For this review, take the finished solid that the model builds, in its own axes (mm). Face numbers are marked on the shaded views. A direction names the side the tool comes from. Give positions to 0.01 mm unless a question says otherwise; leave off trailing zeros. Loops run counter-clockwise (first coordinate to the right, second up) from the corner with the lowest first, then second, coordinate; pieces in that order, holes last. Notation, with made-up numbers: (41.25, 3.5) - (62.25, 3.5) arc R20 cw to (62.25, 10.5) - close; hole circle Ø7 at (39, 1.25). An arc over 180 degrees is marked (long way). Answer as CSV lines item,"result".
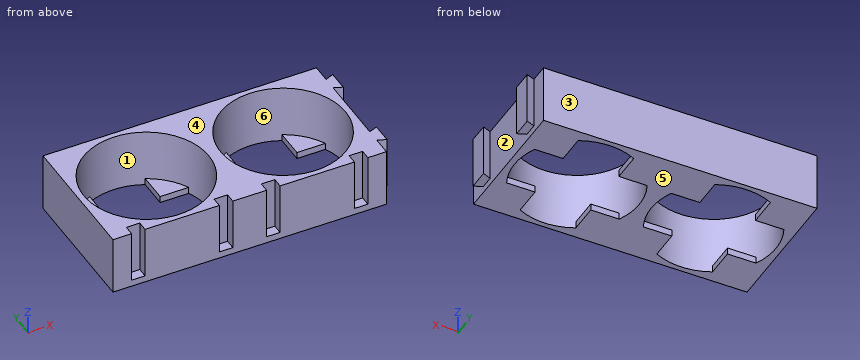
from build123d import *

# Parameters (mm, degrees)
SKETCH1_W           = 40.5
SKETCH1_H           = 20
SKETCH1_R           = 9.25
BOSS_EXTRUDE1_DEPTH = 8.8
SKETCH2_W           = 2
SKETCH2_H           = 7.8
CUT_EXTRUDE1_DEPTH  = 1.5
BOSS_EXTRUDE2_DEPTH = 1


with BuildPart() as part:
    # Sketch1 → Boss-Extrude1 (new body)
    with BuildSketch(Plane.XY):
        Rectangle(SKETCH1_W, SKETCH1_H)
        with Locations((-10.125, 0)):
            Circle(SKETCH1_R, mode=Mode.SUBTRACT)
        with Locations((10.125, 0)):
            Circle(SKETCH1_R, mode=Mode.SUBTRACT)
    extrude(amount=BOSS_EXTRUDE1_DEPTH)

    # Sketch2 → Cut-Extrude1 (cut)
    with BuildSketch(Plane.XZ.offset(10)):
        with Locations((-16.5, 4.9)):
            Rectangle(SKETCH2_W, SKETCH2_H)
        with Locations((-3.5, 4.9)):
            Rectangle(SKETCH2_W, SKETCH2_H)
        with Locations((3.5, 4.9)):
            Rectangle(SKETCH2_W, SKETCH2_H)
        with Locations((16.5, 4.9)):
            Rectangle(SKETCH2_W, SKETCH2_H)
    extrude(amount=-CUT_EXTRUDE1_DEPTH, mode=Mode.SUBTRACT)

    # Sketch3 → Boss-Extrude2 (add)
    with BuildSketch(Plane(origin=(0, 0, 0), x_dir=(-1, 0, 0), z_dir=(0, 0, -1))):
        with BuildLine():
            Line((-14.25, 4), (-14.25, 8.279304017))
            ThreePointArc((-14.25, 8.279304017), (-16.714745453, 6.491360016), (-18.465413659, 4))
            Line((-18.465413659, 4), (-14.25, 4))
        make_face()
        with BuildLine():
            Line((-6, 4), (-1.784586341, 4))
            ThreePointArc((-1.784586341, 4), (-3.535254547, 6.491360016), (-6, 8.279304017))
            Line((-6, 8.279304017), (-6, 4))
        make_face()
        with BuildLine():
            ThreePointArc((-6, -8.279304017), (-3.535254547, -6.491360016), (-1.784586341, -4))
            Line((-1.784586341, -4), (-6, -4))
            Line((-6, -4), (-6, -8.279304017))
        make_face()
        with BuildLine():
            Line((-14.25, -4), (-18.465413659, -4))
            ThreePointArc((-18.465413659, -4), (-16.714745453, -6.491360016), (-14.25, -8.279304017))
            Line((-14.25, -8.279304017), (-14.25, -4))
        make_face()
        with BuildLine():
            Line((1.784586341, 4), (6, 4))
            Line((6, 4), (6, 8.279304017))
            ThreePointArc((6, 8.279304017), (3.535254547, 6.491360016), (1.784586341, 4))
        make_face()
        with BuildLine():
            ThreePointArc((18.465413659, 4), (16.714745453, 6.491360016), (14.25, 8.279304017))
            Line((14.25, 8.279304017), (14.25, 4))
            Line((14.25, 4), (18.465413659, 4))
        make_face()
        with BuildLine():
            Line((14.25, -4), (14.25, -8.279304017))
            ThreePointArc((14.25, -8.279304017), (16.714745453, -6.491360016), (18.465413659, -4))
            Line((18.465413659, -4), (14.25, -4))
        make_face()
        with BuildLine():
            Line((6, -4), (1.784586341, -4))
            ThreePointArc((1.784586341, -4), (3.535254547, -6.491360016), (6, -8.279304017))
            Line((6, -8.279304017), (6, -4))
        make_face()
    extrude(amount=-BOSS_EXTRUDE2_DEPTH)

    # Sketch4 → Loft1 section 0
    with BuildSketch(Plane(origin=(20.25, 0, 0), x_dir=(0, 0, -1), z_dir=(1, 0, 0))):
        with BuildLine():
            Line((-8.8, 7.25), (-1, 7.25))
            Line((-1, 7.25), (-1, 5.25))
            Line((-1, 5.25), (-8.8, 5.25))
            Line((-8.8, 5.25), (-8.8, 7.25))
        make_face()
    # Sketch5 → Loft1 section 1
    with BuildSketch(Plane(origin=(21.5, 0, 0), x_dir=(0, 0, -1), z_dir=(1, 0, 0))):
        with BuildLine():
            Line((-8.8, 7.75), (-1, 7.75))
            Line((-1, 7.75), (-1, 4.75))
            Line((-1, 4.75), (-8.8, 4.75))
            Line((-8.8, 4.75), (-8.8, 7.75))
        make_face()
    loft()

    # Sketch4<3> → Loft2 section 0
    with BuildSketch(Plane(origin=(20.25, 0, 0), x_dir=(0, 0, -1), z_dir=(1, 0, 0))):
        with BuildLine():
            Line((-8.8, -5.25), (-1, -5.25))
            Line((-1, -5.25), (-1, -7.25))
            Line((-1, -7.25), (-8.8, -7.25))
            Line((-8.8, -7.25), (-8.8, -5.25))
        make_face()
    # Sketch5<3> → Loft2 section 1
    with BuildSketch(Plane(origin=(21.5, 0, 0), x_dir=(0, 0, -1), z_dir=(1, 0, 0))):
        with BuildLine():
            Line((-8.8, -4.75), (-1, -4.75))
            Line((-1, -4.75), (-1, -7.75))
            Line((-1, -7.75), (-8.8, -7.75))
            Line((-8.8, -7.75), (-8.8, -4.75))
        make_face()
    loft()


solid = part.part
1) Machinability: for the marked faces 5 and 6, which of the approach directions +Z, -Z, +X, -X, +Y, -Y give a long, thin tool a straight path to every point of the face, cutting with its end or side? Answer none if there is none.
From the geometry:
face 5,"-Z, +X, -X, +Y, -Y"
face 6,"+Z"
2) Wall thickness on line 1 (X direction, y = 0, z = 4) (3 decimals); line 2 (Y direction, x = -17.5, z = 0.75); line 3 (Y direction, x = 10, z = 4.5): over which ranges is each line inside the solid? List them lowest first. Write a range as from..to.
From the geometry:
line 1,"x = -20.25..-19.375, -0.875..0.875, 19.375..20.25"
line 2,"y = -10..-4, 4..10"
line 3,"y = -10..-9.25, 9.25..10"
3) Consider section B-B on z = 5. Count the separate pieces of the cut face and the enclosed holes in it, and give its area (3 significant figures).
From the geometry:
separate pieces,"1"
enclosed holes,"2"
area,"267 mm^2"
4) Consider section D-D on x = 7. Write out the cut boundary in (y, z), and give its area (3 significant figures).
From the geometry:
outline,"(-10, 0) - (-8.71, 0) - (-8.71, 8.8) - (-10, 8.8) - close; (8.71, 0) - (10, 0) - (10, 8.8) - (8.71, 8.8) - close"
area,"22.8 mm^2"
5) Consider section C-C on x = 11.5. Write out the cut boundary in (y, z).
From the geometry:
outline,"(-10, 0) - (-9.15, 0) - (-9.15, 8.8) - (-10, 8.8) - close; (9.15, 0) - (10, 0) - (10, 8.8) - (9.15, 8.8) - close"
6) Consider section A-A on y = 0. Write out the cut boundary in (x, z) (3 decimals).
From the geometry:
outline,"(-20.25, 0) - (-19.375, 0) - (-19.375, 8.8) - (-20.25, 8.8) - close; (-0.875, 0) - (0.875, 0) - (0.875, 8.8) - (-0.875, 8.8) - close; (19.375, 0) - (20.25, 0) - (20.25, 8.8) - (19.375, 8.8) - close"
7) Insertion check: P1, Ø1.2, axis at y = -9, z = 5, coming from the +X side. The pin has a flat end and moves straight along its axis. Give the tip position at first contact, or say it passes through.
From the geometry:
P1,"stops at x = 20.25"
8) Draft analysis for pull direction Y (two halves, no side actions). For the marked faces 1, 2, 3 and 4, state which applies: pulls with the +Y half, pulls with the -Y half, needs draft (parallel to the pull), parting line crosses it, or undercut.
From the geometry:
face 1,"undercut"
face 2,"undercut"
face 3,"pulls with the +Y half"
face 4,"needs draft"
